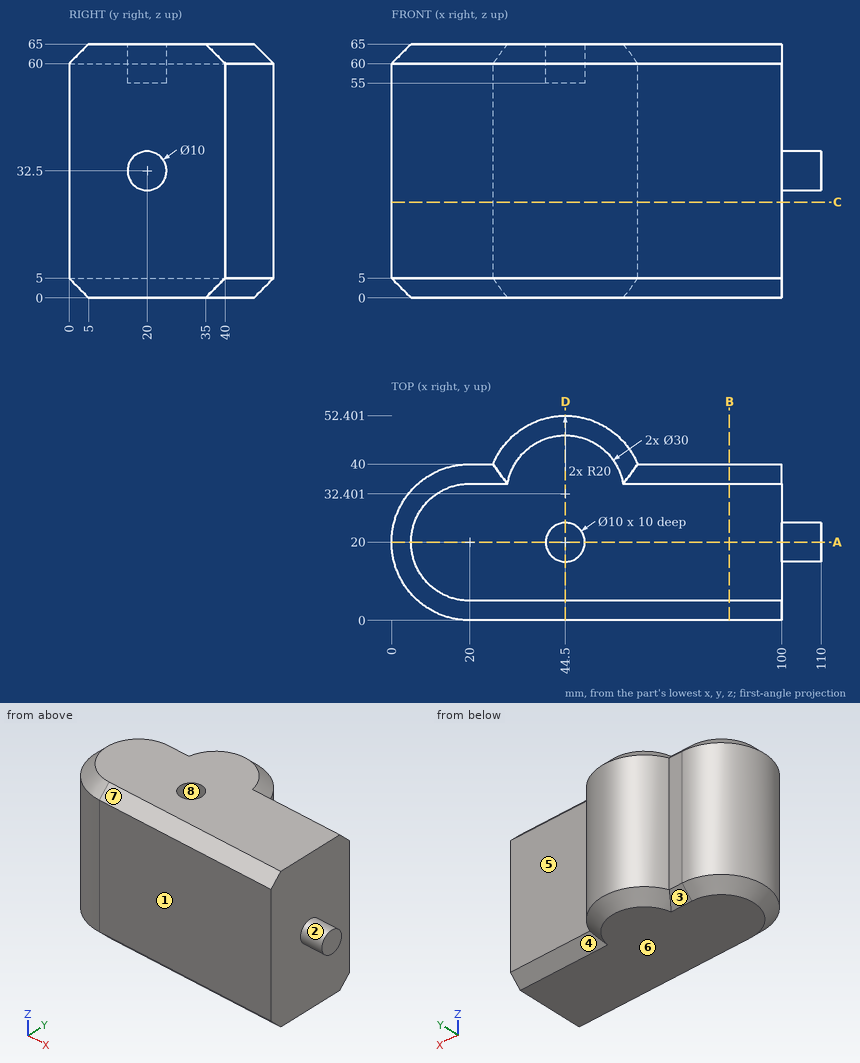
Answer from the drawing. Dimensions are ordinates in mm from the lowest x, y and z of the part. A direction names the side the tool comes from. Coordinates: 2 decimals unless noted, no trailing zeros. Write each loop counter-clockwise with the first axis right and the second up, starting at its lowest first coordinate (ties: lowest second). Pieces come first, ordered by that corner, then holes. Notation, with made-up numbers: M -16,43.5 L 14,43.5 A9 ccw 14,47.5 Z; hole C -16.5,52 d5. An arc over 180 degrees is marked long. Use one line per item in the form item = value. Start each with the question number.
1. Straight lines are drawn through the part: probe 1 along Y at (x, z) = (44, 58) (1 decimal); probe 2 along X at (y, z) = (21, 29.5) (1 decimal); probe 3 along Y at (x, z) = (97.5, 42.5). For each, find the intervals that lie inside material, in ascending order. Write a range as from..to.
2. The part is cut by section D-D (x = 44.5). Give the vertices of the cut face in (y, z).
3. A tool of negligible diameter and unlimited length cuts with its end or side. For the marked faces 1, 2, 3, 4 and 5, from which of +Z, -Z, +X, -X, +Y, -Y can it reach the whole face along a straight path? Write none if from no direction.
4. The part is cut by section C-C (z = 24.5). Give the vertices of the cut face in (x, y).
5. Each of these flat-tipped pins is pushed along its axis until it touches: P1, Ø8, axis at y = 36.5, z = 56, coming from the +X side; P2, Ø1.5, axis at x = 24, y = 37, coming from the +Z side; P3, Ø1.5, axis at x = 33, z = 48, coming from the +Y side (1 decimal). Where does it stop, or does it pass through?
6. The part is cut by section A-A (y = 20). Give the vertices of the cut face in (x, z), plus the area to 4 significant figures.
7. The mould has two halves that part along Y. Classify the marked faces 6, 7 and 8: released by +Y, released by -Y, zero draft, split by the parting line, or undercut.
8. The part is cut by section B-B (x = 86.5). Give the vertices of the cut face in (y, z).
Evaluation:
q1.probe_1 = 0..15, 25..52.4
q1.probe_2 = 0..110
q1.probe_3 = 0..40
q2.outline = M 0,5 L 5,0 L 47.4,0 L 52.4,5 L 52.4,60 L 47.4,65 L 25,65 L 25,55 L 15,55 L 15,65 L 5,65 L 0,60 Z
q3.face_1 = +Z, -Z, +X, -X, -Y
q3.face_2 = +X
q3.face_3 = -Z, -X, +Y
q3.face_4 = -Z, +X, +Y
q3.face_5 = +Z, -Z, +X, +Y
q4.outline = M 20,0 L 100,0 L 100,40 L 63,40 A20 ccw 26,40 L 20,40 A20 ccw Z
q5.P1 = 100
q5.P2 = 63.75
q5.P3 = 49.3
q6.outline = M 0,5 L 5,0 L 100,0 L 100,27.5 L 110,27.5 L 110,37.5 L 100,37.5 L 100,65 L 49.5,65 L 49.5,55 L 39.5,55 L 39.5,65 L 5,65 L 0,60 Z
q6.area = 6,475 mm^2
q7.face_6 = zero draft
q7.face_7 = released by -Y
q7.face_8 = undercut
q8.outline = M 0,5 L 5,0 L 35,0 L 40,5 L 40,60 L 35,65 L 5,65 L 0,60 Z
